Source: CAD feature listing. Evaluate the final solid. Frame: model axes, mm. Face numbers are marked on the shaded views. A direction names the side the tool comes from. Coordinates: 2 decimals unless noted, no trailing zeros. Order: outer loops, then holes, each group sorted by start corner. A loop starts at its lowest first (then second) coordinate and runs counter-clockwise, first axis right, second up.
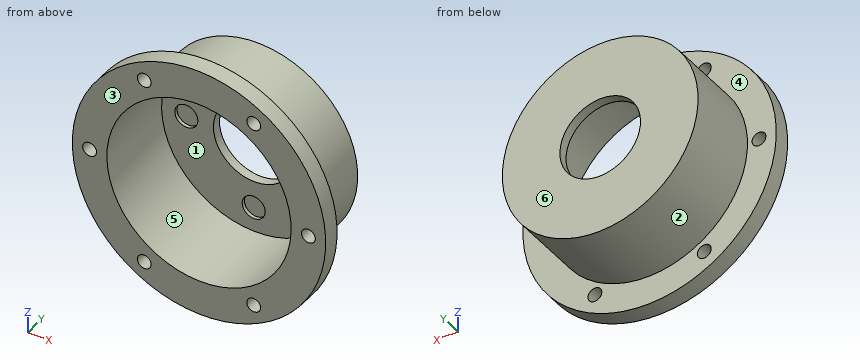
```python
from build123d import *

# Parameters (mm, degrees)
SKETCH2_R                  = 35
CUT_EXTRUDE1_DEPTH         = 8
F_12_0_12_DIAMETER_HOLE1_D = 12
SKETCH7_R                  = 10
CUT_EXTRUDE2_DEPTH         = 3


with BuildPart() as part:
    # Sketch1 → Revolve1 (revolve)
    with BuildSketch(Plane.XY, mode=Mode.PRIVATE) as revolve1_sk:
        Polygon((-80, 72), (0, 72), (0, 80), (-85, 80), (-85, 15), (-110, 15), (-110, 0), (-80, 0), align=None)
    revolve(revolve1_sk.sketch.rotate(Axis((0, 0, 0), (0, 1, 0)), 270), axis=Axis((0, 0, 0), (0, 1, 0)))

    # Sketch2 → Cut-Extrude1 (cut)
    with BuildSketch(Plane(origin=(0, 80, 0), x_dir=(1, 0, 0), z_dir=(0, 1, 0))):
        with Locations(Location((0, 0, 0), (0, 0, 270))):
            Circle(SKETCH2_R)
    extrude(amount=-CUT_EXTRUDE1_DEPTH, mode=Mode.SUBTRACT)

    # Ø12.0 (12) Diameter Hole1 (through all)
    with Locations(Plane(origin=(0, 15, 0), x_dir=(1, 0, 0), z_dir=(0, 1, 0))):
        with Locations((-47.5, -82.27241336), (-95, 0), (-47.5, 82.27241336), (47.5, 82.27241336), (95, 0), (47.5, -82.27241336)):
            Hole(F_12_0_12_DIAMETER_HOLE1_D / 2)

    # Sketch7 → Cut-Extrude2 (cut)
    with BuildSketch(Plane.XZ.offset(-72)):
        with Locations(Location((0, 58.5, 0), (0, 0, 270))):
            Circle(SKETCH7_R)
        with Locations(Location((58.5, 0, 0), (0, 0, 270))):
            Circle(SKETCH7_R)
        with Locations(Location((0, -58.5, 0), (0, 0, 270))):
            Circle(SKETCH7_R)
        with Locations(Location((-58.5, 0, 0), (0, 0, 270))):
            Circle(SKETCH7_R)
    extrude(amount=-CUT_EXTRUDE2_DEPTH, mode=Mode.SUBTRACT)


solid = part.part
```
Q1. Pull-direction query (X, two-part tool) for the marked faces 1, 2 and 3; classes: pulls with the +X half, pulls with the -X half, needs draft (parallel to the pull), parting line crosses it, or undercut.
Solutions:
face 1: undercut
face 2: parting line crosses it
face 3: needs draft
Q2. Section query A-A on x = 0. Output: boundary loops of the cut face in (y, z), plus the area to 3 significant figures.
Solutions:
outline: (0, -110) - (15, -110) - (15, -85) - (80, -85) - (80, -35) - (72, -35) - (72, -48.5) - (75, -48.5) - (75, -68.5) - (72, -68.5) - (72, -80) - (0, -80) - close; (0, 80) - (72, 80) - (72, 68.5) - (75, 68.5) - (75, 48.5) - (72, 48.5) - (72, 35) - (80, 35) - (80, 85) - (15, 85) - (15, 110) - (0, 110) - close
area: 2,150 mm2
Q3. Section query B-B on z = -3. Give the number of separate pieces and of enclosed holes in the cut face, plus the area to 3 significant figures.
Solutions:
separate pieces: 4
enclosed holes: 0
area: 1,850 mm2
Q4. Section query D-D on x = -58.5. Output: boundary loops of the cut face in (y, z), plus the area to 3 significant figures.
Solutions:
outline: (0, -93.15) - (15, -93.15) - (15, -61.67) - (80, -61.67) - (80, 61.67) - (15, 61.67) - (15, 93.15) - (0, 93.15) - (0, 54.57) - (72, 54.57) - (72, 10) - (75, 10) - (75, -10) - (72, -10) - (72, -54.57) - (0, -54.57) - close
area: 2,890 mm2
Q5. Material intervals for line 1 along X through (y, z) = (74, 0); line 2 along Z through (x, y) = (-47.5, 4); line 3 along Z through (x, y) = (-52, 11), sorted ascending.
Solutions:
line 1: x = -85 to -68.5, -48.5 to -35, 35 to 48.5, 68.5 to 85
line 2: z = -99.22 to -88.27, -76.27 to -64.37, 64.37 to 76.27, 88.27 to 99.22
line 3: z = -96.93 to -86.24, -78.3 to -60.79, 60.79 to 78.3, 86.24 to 96.93
Q6. Section query C-C on y = 9.5. Output: boundary loops of the cut face in (x, z).
Solutions:
outline: circle Ø220 at (0, 0); hole circle Ø12 at (-95, 0); hole circle Ø160 at (0, 0); hole circle Ø12 at (-47.5, -82.27); hole circle Ø12 at (-47.5, 82.27); hole circle Ø12 at (47.5, -82.27); hole circle Ø12 at (47.5, 82.27); hole circle Ø12 at (95, 0)
Q7. Pin query (flat end, axial travel): P1, Ø1.5, axis at x = 45.5, y = 58, coming from the +Z side; P2, Ø6, axis at x = 0, z = 60.5, coming from the -Y side; P3, Ø10, axis at x = -74, y = 31, coming from the +Z side. Return the tip coordinate at first contact, or that it passes through.
Solutions:
P1: stops at z = 72.27
P2: stops at y = 75
P3: stops at z = 49.64
Q8. Set-up query: the marked faces 4, 5 and 6. Return all of +Z, -Z, +X, -X, +Y, -Y with unobstructed straight access to the full face (end or side cutting, diameter ignored); none if empty.
Solutions:
face 4: +Y
face 5: -Y
face 6: +Z, -Z, +X, -X, +Y
